Geometry: see drawing. Coordinates: mm, zero at the bounding-box minimum. A direction names the side the tool comes from. Round coordinates to 2 decimals unless told otherwise and drop trailing zeros. Write each loop counter-clockwise with the first axis right and the second up, starting at its lowest first coordinate (ties: lowest second). Pieces come first, ordered by that corner, then holes. Notation, with made-up numbers: (62, -32) -> (86, -32) arc R30 cw to (86, 7) -> close; hole circle Ø2 at (18, -39). An arc over 180 degrees is marked (long way). Write item = value, one per line. Start each with the question number.
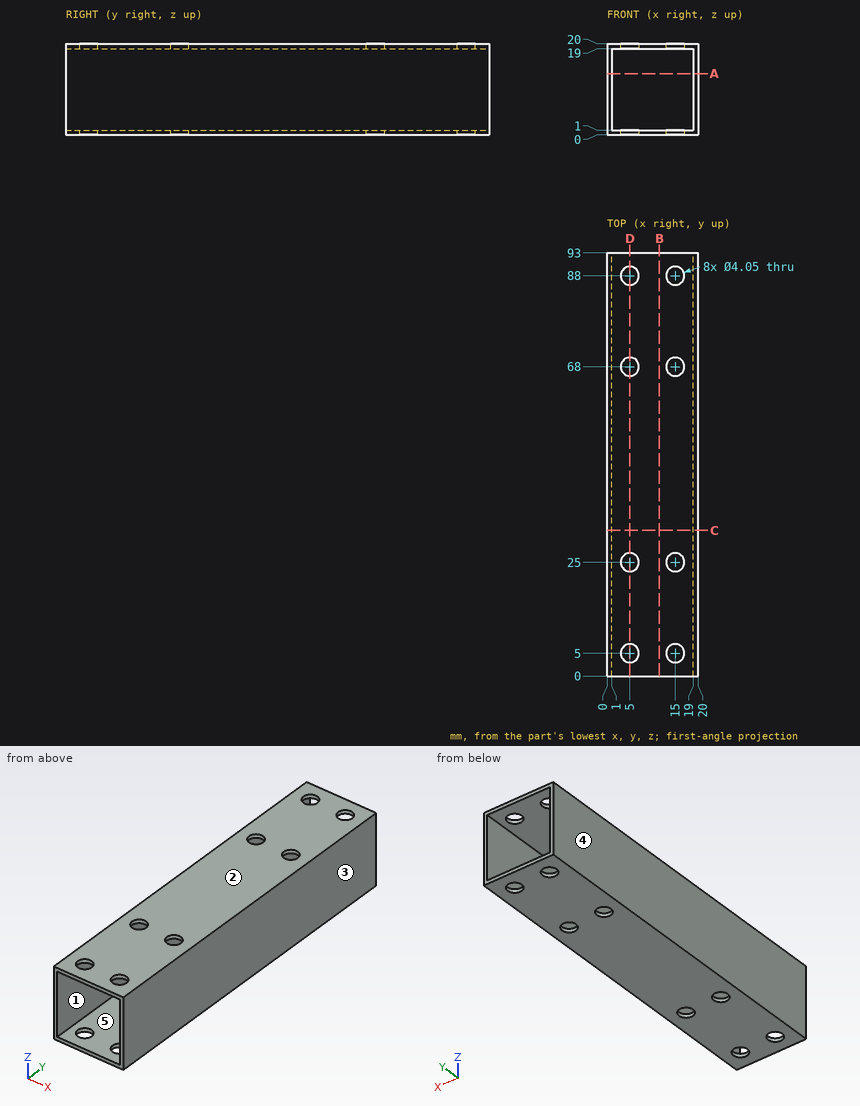
1. Section B-B (x = 11.5). Output: boundary loops of the cut face in (y, z).
2. Line query: line 1 along Y through (x, z) = (15, 19.8) (3 decimals); line 2 along Z through (x, y) = (16.75, 56). Output: solid intervals per line, ascending.
3. Section C-C (y = 32). Output: boundary loops of the cut face in (x, z).
4. Section A-A (z = 13.5). Output: boundary loops of the cut face in (x, y).
5. Mould query, pull axis X, two halves, no side actions, for the marked faces 3, 4 and 5. Classes: pulls with the +X half, pulls with the -X half, needs draft (parallel to the pull), parting line crosses it, or undercut.
6. Reachability of the marked faces 1 and 2 from +Z, -Z, +X, -X, +Y, -Y: full face, straight path, thin tool, end or side. Return the list, or none.
7. Section D-D (x = 5). State how many separate pieces and enclosed holes the cut face has, then the cut area to 3 significant figures.
8. Pin query (flat end, axial travel): P1, Ø3, axis at x = 17, y = 41.5, coming from the -Z side; P2, Ø3.5, axis at x = 5, y = 25, coming from the +Z side. Return the tip coordinate at first contact, or that it passes through.
Check sheet entries:
q1.outline = (0, 0) -> (93, 0) -> (93, 1) -> (0, 1) -> close; (0, 19) -> (93, 19) -> (93, 20) -> (0, 20) -> close
q2.line_1 = 0 to 2.975, 7.025 to 22.975, 27.025 to 65.975, 70.025 to 85.975, 90.025 to 93
q2.line_2 = 0 to 1, 19 to 20
q3.outline = (0, 0) -> (20, 0) -> (20, 20) -> (0, 20) -> close; hole (1, 1) -> (19, 1) -> (19, 19) -> (1, 19) -> close
q4.outline = (0, 0) -> (1, 0) -> (1, 93) -> (0, 93) -> close; (19, 0) -> (20, 0) -> (20, 93) -> (19, 93) -> close
q5.face_3 = pulls with the +X half
q5.face_4 = pulls with the -X half
q5.face_5 = undercut
q6.face_1 = +Y, -Y
q6.face_2 = +Z, +X, -X, +Y, -Y
q7.separate_pieces = 10
q7.enclosed_holes = 0
q7.area = 154 mm2
q8.P1 = 0
q8.P2 = through
